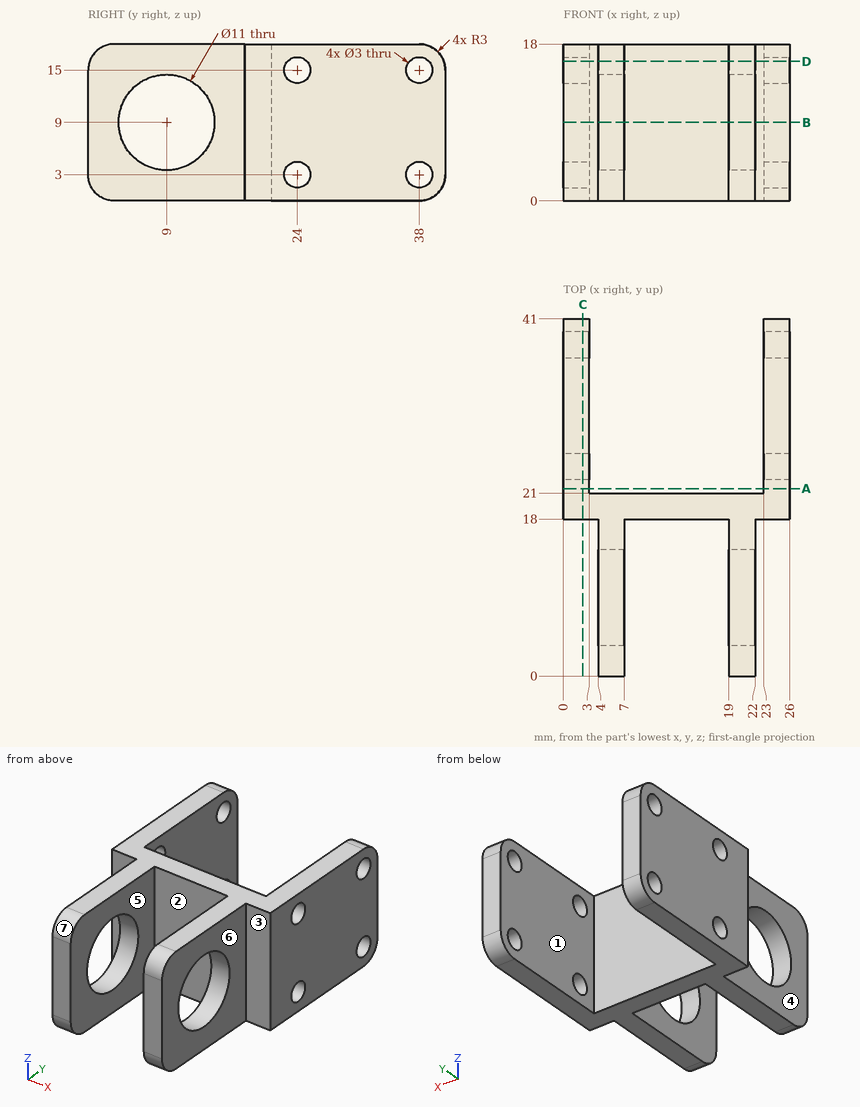
Geometry: see drawing. Coordinates: mm, zero at the bounding-box minimum. A direction names the side the tool comes from. Round coordinates to 2 decimals unless told otherwise and drop trailing zeros. Write each loop counter-clockwise with the first axis right and the second up, starting at its lowest first coordinate (ties: lowest second). Pieces come first, ordered by that corner, then holes.
Item 1: Section query B-B (z = 9). Return loops of the section in (x, y), plus the area to 3 significant figures.
Item 2: Mould query, pull axis X, two halves, no side actions, for the marked faces 5, 6 and 7. Classes: +X half, -X half, draft (parallel to the pull), parting line (faces both ways), or undercut.
Item 3: Section query D-D (z = 16). Give the number of separate pieces and of enclosed holes in the cut face, plus the area to 3 significant figures.
Item 4: Section query C-C (x = 2.25). Return loops of the section in (y, z).
Item 5: Material intervals for L1, parallel to Y at x = 1, z = 15; L2, parallel to X at y = 8.5, z = 1; L3, parallel to X at y = 31.5, z = 1.25, sorted ascending.
Item 6: Section query A-A (y = 21.5). Return loops of the section in (x, z).
Item 7: Set-up query: the marked faces 1, 2, 3 and 4. Return all of +Z, -Z, +X, -X, +Y, -Y with unobstructed straight access to the full face (end or side cutting, diameter ignored); none if empty.
Item 8: Pin query (flat end, axial travel): P1, Ø5.5, axis at y = 7.5, z = 5, coming from the -X side; P2, Ø1.5, axis at x = 22, y = 28, coming from the +Z side; P3, Ø4.5, axis at x = 1.5, z = 5.5, coming from the -Y side; P4, Ø5.5, axis at y = 6.5, z = 11.5, coming from the +X side. Return the tip coordinate at first contact, or that it passes through.
Completed:
1. outline: (0, 18) - (4, 18) - (4, 14.5) - (7, 14.5) - (7, 18) - (19, 18) - (19, 14.5) - (22, 14.5) - (22, 18) - (26, 18) - (26, 41) - (23, 41) - (23, 21) - (3, 21) - (3, 41) - (0, 41) - close; (4, 0) - (7, 0) - (7, 3.5) - (4, 3.5) - close; (19, 0) - (22, 0) - (22, 3.5) - (19, 3.5) - close
1. area: 240 mm2
2. face 5: undercut
2. face 6: +X half
2. face 7: draft
3. separate pieces: 5
3. enclosed holes: 0
3. area: 277 mm2
4. outline: (18, 0) - (38, 0) arc R3 ccw to (41, 3) - (41, 15) arc R3 ccw to (38, 18) - (18, 18) - close; hole circle Ø3 at (24, 3); hole circle Ø3 at (24, 15); hole circle Ø3 at (38, 3); hole circle Ø3 at (38, 15)
5. L1: y = 18 to 22.5, 25.5 to 36.5, 39.5 to 41
5. L2: x = 4 to 7, 19 to 22
5. L3: x = 0 to 3, 23 to 26
6. outline: (0, 0) - (3, 0) - (3, 18) - (0, 18) - close; (23, 0) - (26, 0) - (26, 18) - (23, 18) - close
7. face 1: +Z, -Z, +Y
7. face 2: +Z, -Z, -Y
7. face 3: +Z, -Z, +X, -Y
7. face 4: +Z, -Z, -X, -Y
8. P1: stops at x = 4
8. P2: passes through
8. P3: stops at y = 18
8. P4: stops at x = 22
